from build123d import *

# Parameters (mm, degrees)
SKETCH_1_R          = 2.1
EXTRUDE_1_DEPTH     = 2
SKETCH_2_R          = 2.1
CUT_EXTRUDE_1_DEPTH = 10
SKETCH_3_W          = 2
SKETCH_3_H          = 182.73
EXTRUDE_2_DEPTH     = 19


with BuildPart() as part:
    # ｽｹｯﾁ1 → ﾎﾞｽ - 押し出し1 (new body)
    with BuildSketch(Plane.XY):
        Polygon((0, 0), (0, 182.73), (83.56, 99.17), (83.56, 0), align=None)
        with Locations((8.132919651, 163.990478631)):
            Circle(SKETCH_1_R, mode=Mode.SUBTRACT)
        with Locations((36.417190898, 135.706207384)):
            Circle(SKETCH_1_R, mode=Mode.SUBTRACT)
        with Locations((64.91002614, 107.428490375)):
            Circle(SKETCH_1_R, mode=Mode.SUBTRACT)
        with Locations((76.06, 74.59)):
            Circle(SKETCH_1_R, mode=Mode.SUBTRACT)
        with Locations((76.06, 24.59)):
            Circle(SKETCH_1_R, mode=Mode.SUBTRACT)
    extrude(amount=EXTRUDE_1_DEPTH)

    # ｽｹｯﾁ2 → ｶｯﾄ - 押し出し1 (cut)
    with BuildSketch(Plane.XY.offset(2)):
        with Locations((21.12, 9.69)):
            Circle(SKETCH_2_R)
        with Locations((61.12, 9.69)):
            Circle(SKETCH_2_R)
    extrude(amount=-CUT_EXTRUDE_1_DEPTH, mode=Mode.SUBTRACT)

    # ｽｹｯﾁ3 → ﾎﾞｽ - 押し出し2 (add)
    with BuildSketch(Plane.ZY):
        with Locations((1, 91.365)):
            Rectangle(SKETCH_3_W, SKETCH_3_H)
    extrude(amount=EXTRUDE_2_DEPTH)


solid = part.part
For this review, take the finished solid that the model builds, in its own axes (mm). Round coordinates to 2 decimals unless told otherwise and drop trailing zeros. Write each loop counter-clockwise with the first axis right and the second up, starting at its lowest first coordinate (ties: lowest second). Pieces come first, ordered by that corner, then holes. Notation, with made-up numbers: (-28.5, 56.25) - (-6.5, 56.25) arc R14 cw to (-6.5, 60.25) - close; hole circle Ø11 at (-23, 20). An arc over 180 degrees is marked (long way). Write item = value, one per line. Start each with the question number.
1. Consider section B-B on x = 76.06. State the section outline as (y, z) points.
2. Draft analysis for pull direction Y (two halves, no side actions). For faces 1 (the face through (64.64, 109.51, 0.99)), 2 (the face through (33, 70, 2)), 3 (the face through (41.2, 141.53, 0.99)), state which applies: released by +Y, released by -Y, zero draft, split by the parting line, or undercut.
3. Consider section A-A on x = 21.12. State the section outline as (y, z) points.
4. Wall thickness on L1, parallel to Y at x = 9.5, z = 1.9; L2, parallel to Y at x = 19.5, z = 1; L3, parallel to Y at x = 76.06, z = 1.1: over which ranges is each line inside the solid? List them lowest first.
5. Consider section C-C on y = 74.59. State the section outline as (x, z) points, plus the area to 3 significant figures.
6. Consider section D-D on z = 1. State the section outline as (x, y) points.
Evaluation:
q1.outline = (0, 0) - (22.49, 0) - (22.49, 2) - (0, 2) - close; (26.69, 0) - (72.49, 0) - (72.49, 2) - (26.69, 2) - close; (76.69, 0) - (106.67, 0) - (106.67, 2) - (76.69, 2) - close
q2.face_1 = undercut
q2.face_2 = zero draft
q2.face_3 = released by +Y
q3.outline = (0, 0) - (7.59, 0) - (7.59, 2) - (0, 2) - close; (11.79, 0) - (161.61, 0) - (161.61, 2) - (11.79, 2) - close
q4.L1 = 0 to 162.4, 165.58 to 173.23
q4.L2 = 0 to 8.35, 11.03 to 163.23
q4.L3 = 0 to 22.49, 26.69 to 72.49, 76.69 to 106.67
q5.outline = (-19, 0) - (73.96, 0) - (73.96, 2) - (-19, 2) - close; (78.16, 0) - (83.56, 0) - (83.56, 2) - (78.16, 2) - close
q5.area = 197 mm2
q6.outline = (-19, 0) - (83.56, 0) - (83.56, 99.17) - (0, 182.73) - (-19, 182.73) - close; hole circle Ø4.2 at (8.13, 163.99); hole circle Ø4.2 at (21.12, 9.69); hole circle Ø4.2 at (36.42, 135.71); hole circle Ø4.2 at (61.12, 9.69); hole circle Ø4.2 at (64.91, 107.43); hole circle Ø4.2 at (76.06, 24.59); hole circle Ø4.2 at (76.06, 74.59)
